Model file for the job. Use its own axes, mm. Face numbers are marked on the shaded views. Round coordinates to 2 decimals unless told otherwise and drop trailing zeros. Answer as a JSON object with one key per item and string values.
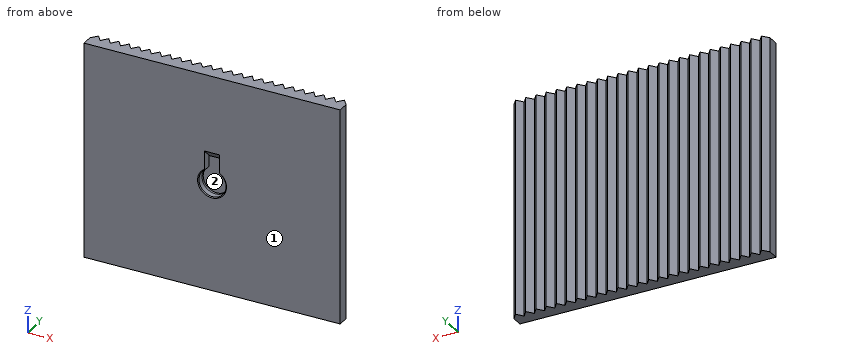
from build123d import *

# Parameters (mm, degrees)
SKETCH1_W           = 58.5
SKETCH1_H           = 49
SKETCH1_R           = 3.1
BOSS_EXTRUDE1_DEPTH = 1.5
BOSS_EXTRUDE2_DEPTH = 49
CUT_EXTRUDE1_DEPTH  = 2
CHAMFER1_SIZE       = 2
CHAMFER2_SIZE       = 0.2


with BuildPart() as part:
    # Sketch1 → Boss-Extrude1 (new body)
    with BuildSketch(Plane(origin=(0, 0, 0), x_dir=(1, 0, 0), z_dir=(0, 1, 0))):
        Rectangle(SKETCH1_W, SKETCH1_H)
        with Locations(Location((0, 0, 0), (0, 0, 270))):
            Circle(SKETCH1_R, mode=Mode.SUBTRACT)
    extrude(amount=BOSS_EXTRUDE1_DEPTH)

    # Sketch2 → Boss-Extrude2 (add)
    with BuildSketch(Plane(origin=(0, 0, -24.5), x_dir=(-1, 0, 0), z_dir=(0, 0, -1))):
        Polygon((-29.25, 1.5), (29.25, 1.5), (29.25, 2.5), (28.08, 4), (26.91, 2.5), (25.74, 4), (24.57, 2.5), (23.4, 4), (22.23, 2.5), (21.06, 4), (19.89, 2.5), (18.72, 4), (17.55, 2.5), (16.38, 4), (15.21, 2.5), (14.04, 4), (12.87, 2.5), (11.7, 4), (10.53, 2.5), (9.36, 4), (8.19, 2.5), (7.02, 4), (5.85, 2.5), (4.68, 4), (3.51, 2.5), (2.34, 4), (1.17, 2.5), (0, 4), (-1.17, 2.5), (-2.34, 4), (-3.51, 2.5), (-4.68, 4), (-5.85, 2.5), (-7.02, 4), (-8.19, 2.5), (-9.36, 4), (-10.53, 2.5), (-11.7, 4), (-12.87, 2.5), (-14.04, 4), (-15.21, 2.5), (-16.38, 4), (-17.55, 2.5), (-18.72, 4), (-19.89, 2.5), (-21.06, 4), (-22.23, 2.5), (-23.4, 4), (-24.57, 2.5), (-25.74, 4), (-26.91, 2.5), (-28.08, 4), (-29.25, 2.5), align=None)
    extrude(amount=-BOSS_EXTRUDE2_DEPTH)

    # Sketch3 → Cut-Extrude1 (cut)
    with BuildSketch(Plane(origin=(0, 0, 0), x_dir=(-1, 0, 0), z_dir=(0, -1, 0))):
        with BuildLine():
            Line((-1.75, -2.558808316), (-1.75, -5))
            Line((-1.75, -5), (1.75, -5))
            Line((1.75, -5), (1.75, -2.558808316))
            ThreePointArc((1.75, -2.558808316), (0, 3.1), (-1.75, -2.558808316))
        make_face()
    extrude(amount=-CUT_EXTRUDE1_DEPTH, mode=Mode.SUBTRACT)

    # Chamfer1
    chamfer1_edges = [part.edges().sort_by_distance(p)[0] for p in [
        (0, 0, 5),
    ]]
    chamfer(chamfer1_edges, length=CHAMFER1_SIZE - 0.0001)  # a hair under: the kernel refuses the full size

    # Chamfer2
    chamfer2_edges = [part.edges().sort_by_distance(p)[0] for p in [
        (0, 0, -3.1),
    ]]
    chamfer(chamfer2_edges, length=CHAMFER2_SIZE)


solid = part.part
1) Two-plate mould, pull along Z, no slides. Class the marked faces 1 and 2: pulls with the +Z half, pulls with the -Z half, needs draft (parallel to the pull), parting line crosses it, or undercut.
Values follow:
{"face 1": "needs draft", "face 2": "undercut"}
2) Probe probe 1 along X at (y, z) = (0.8, 0); probe 2 along Z at (x, y) = (0, 1.1); probe 3 along Z at (x, y) = (-2, 1.9). List the from-to ranges inside material, lowest first.
Values follow:
{"probe 1": "-29.25 to -3.1, 3.1 to 29.25", "probe 2": "-24.5 to -3.1, 5.9 to 24.5", "probe 3": "-24.5 to -2.37, 2.37 to 24.5"}
3) Drop flat-ended pins along their axis: P1, Ø2, axis at x = 7, z = 18.5, coming from the -Y side; P2, Ø8, axis at x = 0, z = 0, coming from the +Y side; P3, Ø1, axis at y = 3.5, z = -0.5, coming from the -X side. Give the stop position or say it passes through.
Values follow:
{"P1": "y = 0", "P2": "y = 4", "P3": "x = -28.86"}
